Could you check a few things on this model? Use its own coordinates, in mm. Face numbers are marked on the shaded views. Give positions to 0.01 mm unless a question says otherwise; leave off trailing zeros. Loops run counter-clockwise (first coordinate to the right, second up) from the corner with the lowest first, then second, coordinate; pieces in that order, holes last. Notation, with made-up numbers: (41, 21.25) - (69, 21.25) arc R27 ccw to (69, 43.25) - close; hole circle Ø9 at (-29, 72.25). An arc over 180 degrees is marked (long way). Write each question's results on one line, items separated by ' | '. Start each with the question number.
1) I want a section at C-C, the plane y = 24.5. Write out the boundary of the cut face in (x, z).
2) I want a section at B-B, the plane z = 7.75. Write out the boundary of the cut face in (x, y).
3) I'm going to push flat-ended pins straight in: pin 1 (10 mm diameter, centred on x = -15, z = 7.5, fed in from -Y); pin 2 (6 mm diameter, centred on x = 23, z = 16.5, fed in from -Y). Where does each tip first touch, or does it pass through?
4) If we mould it in two halves opening along X, with no side actions, what happens to the marked faces 1, 2 and 3? For each: +X half, -X half, draft (parallel to the pull), parting line (faces both ways), or undercut.
5) I want a section at D-D, the plane x = 0. Write out the boundary of the cut face in (y, z).
6) I want a section at A-A, the plane y = 4. Write out the boundary of the cut face in (x, z).
7) If I drill on probe 1 along X at (y, z) = (5, 15.25); probe 2 along X at (y, z) = (26, 13.5); probe 3 along Y at (x, z) = (-20, 6.5), over which ranges is the centre line in solid material (lowest first)? Write a range as [from, to].
Autodesk Inventor part; units mm, degrees
ref_plane "YZ Plane" through (0, 0, 0) normal (1, 0, 0) x (0, 1, 0)
ref_plane "XZ Plane" through (0, 0, 0) normal (0, 1, 0) x (-1, 0, 0)
ref_plane "XY Plane" through (0, 0, 0) normal (0, 0, 1) x (1, 0, 0)
sketch "Sketch13" plane through (0, 0, 0) normal (0, 0, 1) x (1, 0, 0)
  line L0 (-50, 50) -> (50, 50)
  line L1 (50, 50) -> (50, 0)
  line L2 (50, 0) -> (-50, 0)
  line L3 (-50, 0) -> (-50, 50)
  line L4 (-50, 50) -> (50, 0) construction
  line L5 (50, 50) -> (-50, 0) construction
  point P0 (0, 0)
  point P1 (0, 25)
  dimension "d42" = 100
  dimension "d43" = 50
extrude "Extrusion11" add sketch "Sketch13" along normal blind 20
sketch "Sketch14" plane through (0, 0, 20) normal (0, 0, 1) x (1, 0, 0)
  circle A0 centre (0, 0) radius 40
  dimension "d46" = 80
extrude "Extrusion12" cut sketch "Sketch14" against normal blind 20
properties part number "fixation_pipe_v01"
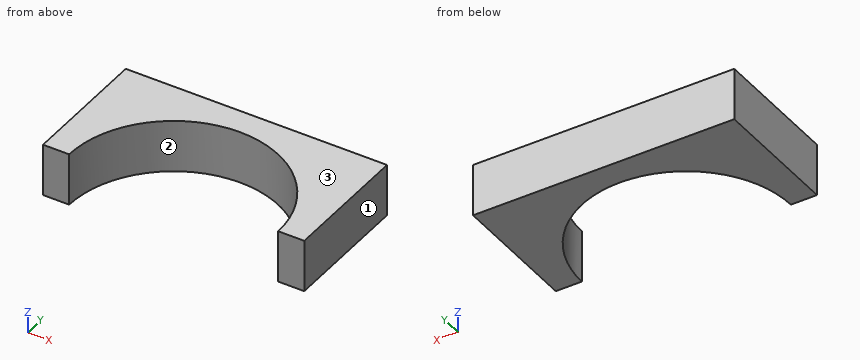
Answers:
1) outline: (-50, 0) - (-31.62, 0) - (-31.62, 20) - (-50, 20) - close; (31.62, 0) - (50, 0) - (50, 20) - (31.62, 20) - close
2) outline: (-50, 0) - (-40, 0) arc R40 cw to (40, 0) - (50, 0) - (50, 50) - (-50, 50) - close
3) pin 1: stops at y = 34.64 | pin 2: stops at y = 30.4
4) face 1: +X half | face 2: undercut | face 3: draft
5) outline: (40, 0) - (50, 0) - (50, 20) - (40, 20) - close
6) outline: (-50, 0) - (-39.8, 0) - (-39.8, 20) - (-50, 20) - close; (39.8, 0) - (50, 0) - (50, 20) - (39.8, 20) - close
7) probe 1: x = [-50, -39.69], [39.69, 50] | probe 2: x = [-50, -30.4], [30.4, 50] | probe 3: y = [34.64, 50]
